Input: part model. Units: mm. Frame: model coordinates. A direction names the side the tool comes from. Give positions to 0.01 mm unless a question says otherwise; leave off trailing zeros. Loops run counter-clockwise (first coordinate to the right, second up) from the corner with the lowest first, then second, coordinate; pieces in that order, holes last.
Autodesk Fusion 360 part; units mm, degrees
sketch "Sketch1" plane through (0, 0, 0) normal (0, 1, 0) x (1, 0, 0)
  line L0 (20, -30) -> (-10, -30)
  line L1 (-10, -30) -> (-10, 0)
  line L2 (0, 0) -> (0, -10)
  line L3 (0, -10) -> (15, 0)
  line L4 (15, 0) -> (25, 0)
  line L5 (20, -30) -> (20, -20)
  line L6 (20, -20) -> (25, -20)
  line L7 (-10, 0) -> (0, 0)
  line L8 (50, 0) -> (50, -10)
  line L9 (60, 0) -> (50, 0)
  line L10 (50, -10) -> (35, 0)
  line L11 (60, -30) -> (60, 0)
  line L12 (30, -30) -> (60, -30)
  line L13 (35, 0) -> (25, 0)
  line L14 (30, -30) -> (30, -20)
  line L15 (30, -20) -> (25, -20)
  point P0 (50, 0)
  dimension "d14" = 30
  dimension "d15" = 30
  dimension "d18" = 10
  dimension "d19" = 15
  dimension "d20" = 10
  dimension "d21" = 15
  dimension "d22" = 10
  dimension "d23" = 5
  dimension "d25" = 10
extrude "Extrude1" add sketch "Sketch1" along normal blind 10
(1) Cut plane D-D (x = 10.5). Return the cut outline in (y, z), and give its area (3 significant figures).
Values follow:
outline: (0, 3) - (10, 3) - (10, 30) - (0, 30) - close
area: 270 mm2
(2) Cut plane C-C (y = 4). Return the cut outline in (x, z), and give its area (3 significant figures).
Values follow:
outline: (-10, 0) - (0, 0) - (0, 10) - (15, 0) - (35, 0) - (50, 10) - (50, 0) - (60, 0) - (60, 30) - (30, 30) - (30, 20) - (20, 20) - (20, 30) - (-10, 30) - close
area: 1,850 mm2
(3) Cut plane B-B (z = 3). Return the cut outline in (x, y), and give its area (3 significant figures).
Values follow:
outline: (-10, 0) - (0, 0) - (0, 10) - (-10, 10) - close; (10.5, 0) - (39.5, 0) - (39.5, 10) - (10.5, 10) - close; (50, 0) - (60, 0) - (60, 10) - (50, 10) - close
area: 490 mm2
(4) Ray query, probe 1 along X at (y, z) = (7.25, 26); probe 2 along X at (y, z) = (8.5, 6.5); probe 3 along X at (y, z) = (1.75, 5.75) (3 decimals). Return the intervals inside material, ascending.
Values follow:
probe 1: x = -10 to 20, 30 to 60
probe 2: x = -10 to 0, 5.25 to 44.75, 50 to 60
probe 3: x = -10 to 0, 6.375 to 43.625, 50 to 60
(5) Cut plane A-A (z = 27.5). Return the cut outline in (x, y).
Values follow:
outline: (-10, 0) - (20, 0) - (20, 10) - (-10, 10) - close; (30, 0) - (60, 0) - (60, 10) - (30, 10) - close
(6) Reachability of faces 1 (the flat face through (45, 5, 30)), 2 (the flat face through (25, 5, 20)), 3 (the flat face through (50, 5, 5)) from +Z, -Z, +X, -X, +Y, -Y: full face, straight path, thin tool, end or side. Return the list, or none.
Values follow:
face 1: +Z, +X, -X, +Y, -Y
face 2: +Z, +Y, -Y
face 3: -Z, +Y, -Y
(7) Pin query (flat end, axial travel): pin 1 Ø4 at (x, y) = (43, 1) entering from -Z. Return the tip coordinate at first contact, or that it passes through.
Values follow:
pin 1: stops at z = 4
